Part model, mm, in its own coordinate system. A direction names the side the tool comes from. Give positions to 0.01 mm unless a question says otherwise; leave off trailing zeros. Order: outer loops, then holes, each group sorted by start corner. A loop starts at its lowest first (then second) coordinate and runs counter-clockwise, first axis right, second up.
1. Drop flat-ended pins along their axis: pin 1 Ø5 at (x, z) = (-6.5, 8) entering from -Y; pin 2 Ø0.6 at (x, z) = (-6.5, 6.5) entering from +Y; pin 3 Ø1 at (x, z) = (-6.5, 7) entering from -Y; pin 4 Ø1 at (x, y) = (0.5, -2.5) entering from +Z. Give the stop position or say it passes through.
2. Slice it at A-A on y = 0. List the corners of the cut face in (x, z), and give its area (4 significant figures).
3. Slice it at D-D on x = -6. List the corners of the cut face in (y, z).
4. Which spindle directions (+Z, -Z, +X, -X, +Y, -Y) get a long thin tool onto all of the face, cutting with end or side? Do faces 4 (the flat face through (0, 6, 21)), 5 (the flat face through (6, 0, 27)), 6 (the flat face through (-6, -2.5, 7)). Say none if no direction does.
5. Slice it at B-B on x = 0. List the corners of the cut face in (y, z), and give its area (3 significant figures).
6. Mould opens along X. For faces 1 (the cylindrical face through (9.237, -3.83, 13.311)), 2 (the flat face through (7, 0, 0)), 3 (the flat face through (0, -7, 21)) say: +X half, -X half, draft (parallel to the pull), parting line (faces both ways), or undercut.
7. Probe line 1 (Y direction, x = 0, z = 8.5); line 2 (X direction, y = 0, z = 9.5); line 3 (Z direction, x = -0.25, y = 8). List the from-to ranges inside material, lowest first.
8. Slice it at C-C on z = 7.75. List the corners of the cut face in (x, y).
from build123d import *

# Parameters (mm, degrees)
SKETCH1_R           = 10
BOSS_EXTRUDE1_DEPTH = 27
SKETCH2_R           = 4
CUT_EXTRUDE1_DEPTH  = 140
SKETCH3_R           = 6
CUT_EXTRUDE2_DEPTH  = 15
SKETCH4_W           = 6
SKETCH4_H           = 6
CUT_EXTRUDE3_DEPTH  = 15
SKETCH5_W           = 3.5796646
SKETCH5_H           = 5
CUT_EXTRUDE4_DEPTH  = 15


with BuildPart() as part:
    # Sketch1 → Boss-Extrude1 (new body)
    with BuildSketch(Plane.XY):
        Circle(SKETCH1_R)
    extrude(amount=BOSS_EXTRUDE1_DEPTH)

    # Sketch2 → Cut-Extrude1 (cut)
    with BuildSketch(Plane.XY.offset(27)):
        Circle(SKETCH2_R)
    extrude(amount=-CUT_EXTRUDE1_DEPTH, mode=Mode.SUBTRACT)

    # Sketch3 → Cut-Extrude2 (cut)
    with BuildSketch(Plane(origin=(0, 0, 0), x_dir=(-1, 0, 0), z_dir=(0, 0, -1))):
        Circle(SKETCH3_R)
    extrude(amount=-CUT_EXTRUDE2_DEPTH, mode=Mode.SUBTRACT)

    # Sketch4 → Cut-Extrude3 (cut, symmetric)
    with BuildSketch(Plane(origin=(0, 0, 0), x_dir=(1, 0, 0), z_dir=(0, 1, 0))):
        with Locations((0, -24)):
            Rectangle(SKETCH4_W, SKETCH4_H)
    extrude(amount=CUT_EXTRUDE3_DEPTH, both=True, mode=Mode.SUBTRACT)

    # Sketch5 → Cut-Extrude4 (cut)
    with BuildSketch(Plane(origin=(0, 0, 0), x_dir=(-1, 0, 0), z_dir=(0, 0, -1))):
        with Locations((5.7101677, 0)):
            Rectangle(SKETCH5_W, SKETCH5_H)
    extrude(amount=-CUT_EXTRUDE4_DEPTH, mode=Mode.SUBTRACT)


solid = part.part
Data:
1. pin 1: stops at y = -9.17
1. pin 2: stops at y = 7.85
1. pin 3: stops at y = -8
1. pin 4: passes through
2. outline: (-10, 0) - (-7.5, 0) - (-7.5, 15) - (-4, 15) - (-4, 27) - (-10, 27) - close; (4, 15) - (6, 15) - (6, 0) - (10, 0) - (10, 27) - (4, 27) - close
2. area: 241.5 mm2
3. outline: (-8, 0) - (-2.5, 0) - (-2.5, 15) - (2.5, 15) - (2.5, 0) - (8, 0) - (8, 27) - (-8, 27) - close
4. face 4: +Z, +Y, -Y
4. face 5: +Z, +X, -X, +Y, -Y
4. face 6: -Z
5. outline: (-10, 0) - (-6, 0) - (-6, 15) - (-4, 15) - (-4, 21) - (-10, 21) - close; (4, 15) - (6, 15) - (6, 0) - (10, 0) - (10, 21) - (4, 21) - close
5. area: 192 mm2
6. face 1: parting line
6. face 2: draft
6. face 3: undercut
7. line 1: y = -10 to -6, 6 to 10
7. line 2: x = -10 to -7.5, 6 to 10
7. line 3: z = 0 to 21
8. outline: circle Ø20 at (0, 0); hole (-7.5, -2.5) - (-5.45, -2.5) arc R6 ccw (long way) to (-5.45, 2.5) - (-7.5, 2.5) - close
